The drawing under review shows one solid part. Ordinate dimensions are in mm from its lowest x, y, z. A direction names the side the tool comes from. Round coordinates to 2 decimals unless told otherwise and drop trailing zeros. Write each loop counter-clockwise with the first axis right and the second up, starting at its lowest first coordinate (ties: lowest second). Pieces come first, ordered by that corner, then holes. Notation, with made-up numbers: (5.25, 35) -> (23.25, 35) arc R15 cw to (23.25, 59) -> close; hole circle Ø2 at (23.5, 23.5). An arc over 180 degrees is marked (long way). Use CSV: the item, a comma, the result in double quotes. Start each with the question number.
1) Wall thickness on probe 1 along Z at (x, y) = (16.5, 10.25); probe 2 along Z at (x, y) = (10, 11); probe 3 along Z at (x, y) = (44.5, 25.25): over which ranges is each line inside the solid? List them lowest first. Write a range as [from, to].
2) For pin 1 Ø4 at (y, z) = (12.5, 48) entering from +X; pin 2 Ø2.5 at (y, z) = (18.5, 6.5) entering from +X; pin 3 Ø2.5 at (x, z) = (36.5, 59.5) entering from -Y, all flat-tipped, find the tip position at first contact; note any pin that passes through.
3) Take a section at D-D, the plane x = 10.5. Give the boundary of the cut face in (y, z), then the cut area to 3 significant figures.
4) Mouldability with a two-part tool opening along Z and no side actions: class the marked faces 5, 6, 7 and 8 as released by +Z, released by -Z, zero draft, split by the parting line, or undercut.
5) Machinability: for the marked faces 1, 2, 3 and 4, which of the approach directions +Z, -Z, +X, -X, +Y, -Y give a long, thin tool a straight path to every point of the face, cutting with its end or side? Answer none if there is none.
6) Take a section at A-A, the plane y = 17. Give the boundary of the cut face in (x, z), then the cut area to 3 significant figures.
7) Take a section at C-C, the plane z = 28.5. Give the boundary of the cut face in (x, y).
8) Take a section at B-B, the plane y = 7.75. Give the boundary of the cut face in (x, z), then the cut area to 3 significant figures.
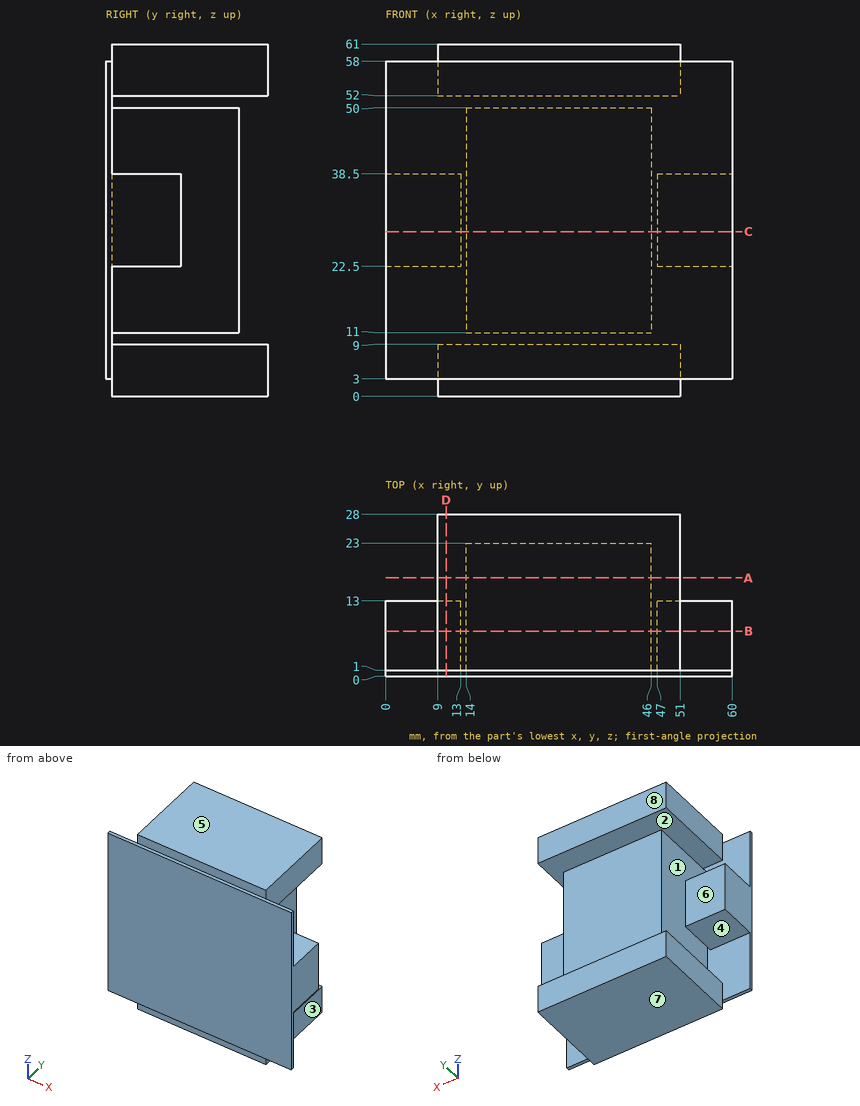
Values found:
1,probe 1,"[0, 9], [11, 50], [52, 61]"
1,probe 2,"[0, 9], [22.5, 38.5], [52, 61]"
1,probe 3,"[0, 9], [52, 61]"
2,pin 1,"x = 46"
2,pin 2,"x = 51"
2,pin 3,"y = 1"
3,outline,"(0, 3) -> (1, 3) -> (1, 0) -> (28, 0) -> (28, 9) -> (1, 9) -> (1, 22.5) -> (13, 22.5) -> (13, 38.5) -> (1, 38.5) -> (1, 52) -> (28, 52) -> (28, 61) -> (1, 61) -> (1, 58) -> (0, 58) -> close"
3,area,"733 mm²"
4,face 5,"released by +Z"
4,face 6,"undercut"
4,face 7,"released by -Z"
4,face 8,"zero draft"
5,face 1,"+Y"
5,face 2,"+X, -X, +Y"
5,face 3,"-Z, +X, +Y"
5,face 4,"-X, +Y"
6,outline,"(9, 0) -> (51, 0) -> (51, 9) -> (9, 9) -> close; (9, 52) -> (51, 52) -> (51, 61) -> (9, 61) -> close; (14, 11) -> (46, 11) -> (46, 50) -> (14, 50) -> close"
6,area,"2,000 mm²"
7,outline,"(0, 0) -> (60, 0) -> (60, 13) -> (47, 13) -> (47, 1) -> (46, 1) -> (46, 23) -> (14, 23) -> (14, 1) -> (13, 1) -> (13, 13) -> (0, 13) -> close"
8,outline,"(0, 22.5) -> (13, 22.5) -> (13, 38.5) -> (0, 38.5) -> close; (9, 0) -> (51, 0) -> (51, 9) -> (9, 9) -> close; (9, 52) -> (51, 52) -> (51, 61) -> (9, 61) -> close; (14, 11) -> (46, 11) -> (46, 50) -> (14, 50) -> close; (47, 22.5) -> (60, 22.5) -> (60, 38.5) -> (47, 38.5) -> close"
8,area,"2,420 mm²"
